Check sheet for the drawn part. Datum: minimum x, y, z corner. Units: mm. A direction names the side the tool comes from. Round coordinates to 2 decimals unless told otherwise and drop trailing zeros. Write each loop counter-clockwise with the first axis right and the second up, starting at its lowest first coordinate (ties: lowest second). Pieces come first, ordered by that corner, then holes. Notation, with made-up numbers: (79, 23) - (93, 23) arc R23 ccw to (93, 46) - close; hole circle Ø1 at (58, 18.5). An arc over 180 degrees is marked (long way). Answer as a JSON object with one key per item and string values. Group by question number.
Item 1: Set-up check for the marked faces 5 and 6: record each of +Z, -Z, +X, -X, +Y, -Y from which the full face is reachable in a straight line by a thin tool's end or side.
Item 2: Gauge pin test, flat ends, axial feed: P1, Ø1, axis at y = 16.5, z = 16.5, coming from the +X side; P2, Ø8, axis at x = 36.5, z = 11.5, coming from the -Y side; P3, Ø1.5, axis at y = 18, z = 8.5, coming from the -X side; P4, Ø3, axis at x = 7.5, z = 5, coming from the +Y side. Record the tip position at first contact, or that the pin passes through.
Item 3: Sectioned sample at B-B on y = 21. Record the boundary of the cut face in (x, z).
Item 4: Thickness scan on line 1 (Y direction, x = 30, z = 17.4); line 2 (Y direction, x = 30, z = 7.75); line 3 (X direction, y = 36.5, z = 6.5). Record the ranges inside material, lowest first.
Item 5: Sectioned sample at C-C on z = 19. Record the boundary of the cut face in (x, y).
Item 6: Sectioned sample at D-D on z = 4. Record the boundary of the cut face in (x, y), plus the area to 3 significant figures.
Item 7: Release check for a two-part mould opening along X. For the marked faces 1, 2, 3 and 4 record: pulls with the +X half, pulls with the -X half, needs draft (parallel to the pull), parting line crosses it, or undercut.
Item 8: Sectioned sample at A-A on x = 30. Record the boundary of the cut face in (y, z), plus the area to 3 significant figures.
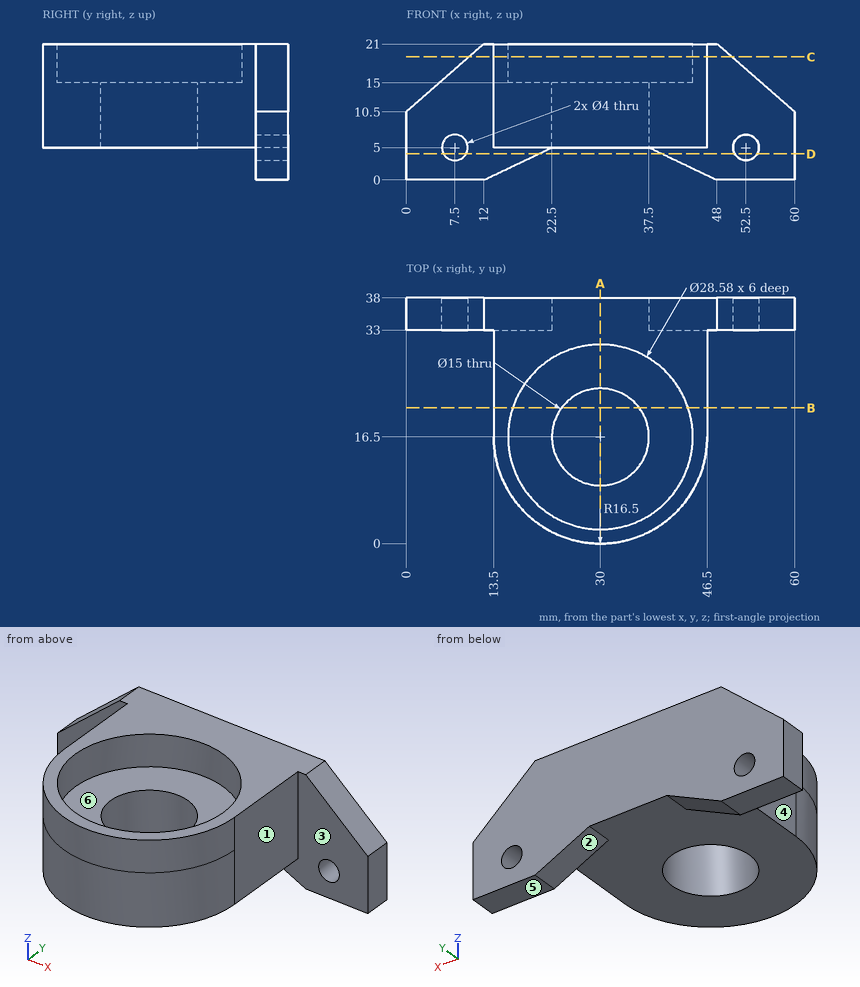
Completed:
{
 "1": {"face 5": "-Z, +X, -X, +Y, -Y", "face 6": "+Z"},
 "2": {"P1": "x = 46.5", "P2": "y = 0.19", "P3": "x = 13.5", "P4": "through"},
 "3": {"outline": "(13.5, 5) - (24, 5) - (24, 15) - (16.44, 15) - (16.44, 21) - (13.5, 21) - close; (36, 5) - (46.5, 5) - (46.5, 21) - (43.56, 21) - (43.56, 15) - (36, 15) - close"},
 "4": {"line 1": "0 to 2.21, 30.79 to 38", "line 2": "0 to 9, 24 to 38", "line 3": "0 to 6.18, 8.82 to 51.18, 53.82 to 60"},
 "5": {"outline": "(9.71, 33) - (13.5, 33) - (13.5, 16.5) arc R16.5 ccw to (46.5, 16.5) - (46.5, 33) - (50.29, 33) - (50.29, 38) - (9.71, 38) - close; hole circle Ø28.58 at (30, 16.5)"},
 "6": {"outline": "(0, 33) - (5.77, 33) - (5.77, 38) - (0, 38) - close; (9.23, 33) - (20.4, 33) - (20.4, 38) - (9.23, 38) - close; (39.6, 33) - (50.77, 33) - (50.77, 38) - (39.6, 38) - close; (54.23, 33) - (60, 33) - (60, 38) - (54.23, 38) - close", "area": "169 mm²"},
 "7": {"face 1": "pulls with the +X half", "face 2": "undercut", "face 3": "needs draft", "face 4": "pulls with the -X half"},
 "8": {"outline": "(0, 5) - (9, 5) - (9, 15) - (2.21, 15) - (2.21, 21) - (0, 21) - close; (24, 5) - (38, 5) - (38, 21) - (30.79, 21) - (30.79, 15) - (24, 15) - close", "area": "287 mm²"}
}
